Check sheet for the modelled part. Datum: model origin and axes. Units: mm. Coordinates: 2 decimals unless noted, no trailing zeros. Write each loop counter-clockwise with the first axis right and the second up, starting at its lowest first coordinate (ties: lowest second). Pieces come first, ordered by that corner, then holes. Notation, with made-up numbers: M 21,6.5 L 61,6.5 A25 cw 61,39.5 Z; hole C 9,77.25 d10. An arc over 180 degrees is marked long. Answer as CSV lines item,"result". Start each with the question number.
Q1. Sectioned sample at B-B, the plane y = -13. Record the cut outline in (x, z) (3 decimals).
Q2. Sectioned sample at C-C, the plane x = 15. Record the cut outline in (y, z), then the cut area to 3 significant figures.
Q3. Sectioned sample at A-A, the plane x = 26. Record the cut outline in (y, z).
Q4. Depth check by flat-ended pin: pin 1 Ø6 at (x, z) = (7.5, -6.5) entering from +Y; pin 2 Ø3 at (y, z) = (-13, -6.275) entering from -X; pin 3 Ø12 at (y, z) = (-17, -8.5) entering from +X; pin 4 Ø8 at (y, z) = (-43.5, -6.5) entering from -X. Enter the tip coordinate at first touch or a pass-through.
Q5. Thickness scan on line 1 along Y through (x, z) = (3.5, -15.75); line 2 along X through (y, z) = (-15.5, -5.5); line 3 along X through (y, z) = (-16, -14). Record the ranges inside material, lowest first. Write a range as from..to.
from build123d import *

# Parameters (mm, degrees)
BOSS_EXTRUDE1_DEPTH = 25.05
SKETCH3_R           = 1.75
CUT_EXTRUDE1_DEPTH  = 73.231514091
SKETCH4_R           = 1.75
CUT_EXTRUDE2_DEPTH  = 73.231514091


with BuildPart() as part:
    # Sketch1 → Boss-Extrude1 (new body)
    with BuildSketch(Plane.XY):
        Polygon((0, 0), (0.254034118, 0), (32.772967712, -56.324445192), (32.518933594, -56.324445192), align=None)
    extrude(amount=-BOSS_EXTRUDE1_DEPTH)

    # Sketch3 → Cut-Extrude1 (cut, through all)
    with BuildSketch(Plane.ZY.offset(4.876016361)):
        with Locations(Location((-18.775, -13, 0), (0, 0, 90))):
            Circle(SKETCH3_R)
        with Locations(Location((-6.275, -13, 0), (0, 0, 90))):
            Circle(SKETCH3_R)
    extrude(amount=-CUT_EXTRUDE1_DEPTH, mode=Mode.SUBTRACT)

    # Sketch4 → Cut-Extrude2 (cut, through all)
    with BuildSketch(Plane(origin=(37.648984073, 0, 0), x_dir=(0, 0, -1), z_dir=(1, 0, 0))):
        with Locations(Location((6.75, -44.449445192, 0), (0, 0, 270))):
            Circle(SKETCH4_R)
        with Locations(Location((19.25, -44.449445192, 0), (0, 0, 270))):
            Circle(SKETCH4_R)
    extrude(amount=-CUT_EXTRUDE2_DEPTH, mode=Mode.SUBTRACT)


solid = part.part
Output:
1,outline,"M 7.506,-25.05 L 7.76,-25.05 L 7.76,-20.525 L 7.506,-20.525 Z; M 7.506,-17.025 L 7.76,-17.025 L 7.76,-8.025 L 7.506,-8.025 Z; M 7.506,-4.525 L 7.76,-4.525 L 7.76,0 L 7.506,0 Z"
2,outline,"M -25.98,-25.05 L -25.54,-25.05 L -25.54,0 L -25.98,0 Z"
2,area,"11.0 mm^2"
3,outline,"M -45.03,-25.05 L -44.59,-25.05 L -44.59,-20.99 A1.75 cw -45.03,-20.9 Z; M -45.03,-17.6 A1.75 cw -44.59,-17.51 L -44.59,-8.49 A1.75 cw -45.03,-8.4 Z; M -45.03,-5.1 A1.75 cw -44.59,-5.01 L -44.59,0 L -45.03,0 Z"
4,pin 1,"stops at y = -7.35"
4,pin 2,"passes through"
4,pin 3,"stops at x = 13.53"
4,pin 4,"stops at x = 22.81"
5,line 1,"y = -6.06..-5.62"
5,line 2,"x = 8.95..9.2"
5,line 3,"x = 9.24..9.49"
